```python
from build123d import *

# Parameters (mm, degrees)
F0_R     = 36.25
F1_DEPTH = 43
F2_R     = 35.25
F3_DEPTH = 39
F5_R     = 36.25
F5_R_2   = 30.25
F6_DEPTH = 2
F7_W     = 7.17
F7_H     = 26
F8_DEPTH = 43.001


with BuildPart() as f1:
    # F0 (on Top) → F1 (new body)
    with BuildSketch(Plane.XY):
        Circle(F0_R)
    extrude(amount=F1_DEPTH)

    # F2 (on face) → F3 (cut)
    with BuildSketch(Plane.XY.offset(43)):
        Circle(F2_R)
    extrude(amount=-F3_DEPTH, mode=Mode.SUBTRACT)

    # F5 (on offset) → F6 (join)
    with BuildSketch(Plane.XY.offset(38)):
        Circle(F5_R)
        Circle(F5_R_2, mode=Mode.SUBTRACT)
    extrude(amount=-F6_DEPTH)

    # F7 (on Top) → F8 (cut, through all)
    with BuildSketch(Plane.XY):
        Rectangle(F7_W, F7_H)
    extrude(amount=F8_DEPTH, mode=Mode.SUBTRACT)


solid = f1.part
```
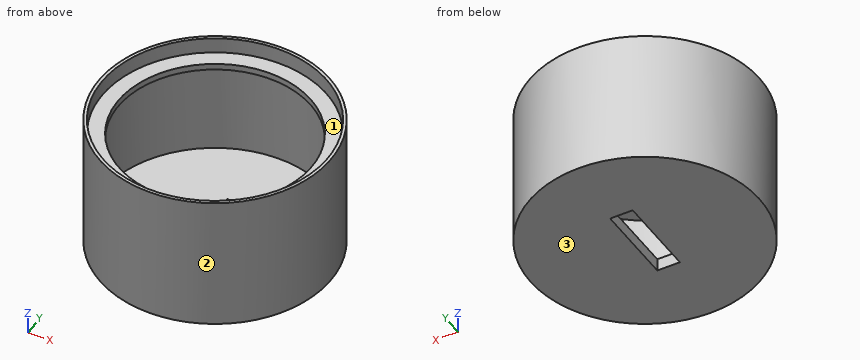
Check sheet for the modelled part. Datum: model origin and axes. Units: mm. Face numbers are marked on the shaded views. Give positions to 0.01 mm unless a question says otherwise; leave off trailing zeros. Loops run counter-clockwise (first coordinate to the right, second up) from the corner with the lowest first, then second, coordinate; pieces in that order, holes last. Notation, with made-up numbers: (9, 58.5) - (29, 58.5) arc R16 cw to (29, 74.5) - close; hole circle Ø7 at (73, -16). An arc over 180 degrees is marked (long way). One line per question, with ' | ' between items. Start each with the question number.
1. Cross-section at D-D, the plane x = -9.5. Enter the section's corners in (y, z), plus the area to 3 significant figures.
2. Cross-section at B-B, the plane y = 0. Enter the section's corners in (x, z) (3 decimals).
3. Cross-section at C-C, the plane z = 18. Enter the section's corners in (x, y).
4. Draft check along X on the marked faces 1, 2 and 3. Enter one of: released by +X, released by -X, zero draft, split by the parting line, or undercut.
5. Material ranges on line 1 along Z through (x, y) = (3, -18.5); line 2 along Z through (x, y) = (30.5, -12.5); line 3 along Y through (x, z) = (21, 6), recorded low to high. Write a range as [from, to].
6. Gauge pin test, flat ends, axial feed: pin 1 Ø21 at (x, y) = (9, 9) entering from +Z; pin 2 Ø1.2 at (y, z) = (-5.5, 2.5) entering from -X; pin 3 Ø6 at (x, y) = (-8.5, 12.5) entering from -Z; pin 4 Ø5 at (y, z) = (-22, 27.5) entering from -X. Record the tip position at first contact, or that the pin passes through.
7. Cross-section at A-A, the plane x = 0. Enter the section's corners in (y, z).
Check result:
1) outline: (-34.98, 0) - (34.98, 0) - (34.98, 43) - (33.95, 43) - (33.95, 38) - (28.72, 38) - (28.72, 36) - (33.95, 36) - (33.95, 4) - (-33.95, 4) - (-33.95, 36) - (-28.72, 36) - (-28.72, 38) - (-33.95, 38) - (-33.95, 43) - (-34.98, 43) - close | area: 382 mm2
2) outline: (-36.25, 0) - (-3.585, 0) - (-3.585, 4) - (-35.25, 4) - (-35.25, 36) - (-30.25, 36) - (-30.25, 38) - (-35.25, 38) - (-35.25, 43) - (-36.25, 43) - close; (3.585, 0) - (36.25, 0) - (36.25, 43) - (35.25, 43) - (35.25, 38) - (30.25, 38) - (30.25, 36) - (35.25, 36) - (35.25, 4) - (3.585, 4) - close
3) outline: circle Ø72.5 at (0, 0); hole circle Ø70.5 at (0, 0)
4) face 1: undercut | face 2: split by the parting line | face 3: zero draft
5) line 1: z = [0, 4] | line 2: z = [0, 4], [36, 38] | line 3: y = [-29.55, -28.31], [28.31, 29.55]
6) pin 1: stops at z = 4 | pin 2: stops at x = -35.92 | pin 3: stops at z = 0 | pin 4: stops at x = -30.56
7) outline: (-36.25, 0) - (-13, 0) - (-13, 4) - (-35.25, 4) - (-35.25, 36) - (-30.25, 36) - (-30.25, 38) - (-35.25, 38) - (-35.25, 43) - (-36.25, 43) - close; (13, 0) - (36.25, 0) - (36.25, 43) - (35.25, 43) - (35.25, 38) - (30.25, 38) - (30.25, 36) - (35.25, 36) - (35.25, 4) - (13, 4) - close
